Geometry check sheet. Reference: the model listing, model coordinates, mm. Face numbers are marked on the shaded views. A direction names the side the tool comes from. Coordinates: 2 decimals unless noted, no trailing zeros. Order: outer loops, then holes, each group sorted by start corner. A loop starts at its lowest first (then second) coordinate and runs counter-clockwise, first axis right, second up. Notation, with made-up numbers: (17.25, -29.5) - (72.25, -29.5) arc R18 ccw to (72.25, -15.5) - close; hole circle Ø1 at (-39, 16). An arc over 180 degrees is marked (long way). One line per item, written item: value. Start each with the question number.
```python
from build123d import *

# Parameters (mm, degrees)
F0_W     = 84
F0_H     = 68
F1_DEPTH = 50
F4_D     = 20
F5_D     = 20
F5_DEPTH = 50


with BuildPart() as f1:
    # F0 (on Top) → F1 (new body)
    with BuildSketch(Plane.XY):
        Polygon((0, 200), (0, 0), (16, 0), (16, 50), (116, 50), (116, 150), (16, 150), (16, 200), align=None)
        with Locations((58, 100)):
            Rectangle(F0_W, F0_H, mode=Mode.SUBTRACT)
    extrude(amount=F1_DEPTH)

    # F4 (through all)
    with Locations(Plane.YZ.offset(16)):
        with Locations((25, 25), (175, 25)):
            Hole(F4_D / 2)

    # F5
    with Locations(Plane.YZ.offset(116)):
        with Locations((100, 25)):
            Hole(F5_D / 2, depth=F5_DEPTH)


solid = f1.part
```
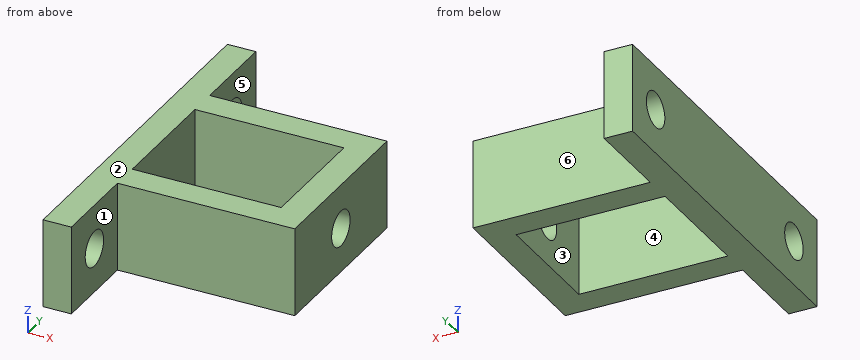
Q1. Cross-section at B-B, the plane x = 91.5. Enter the section's corners in (y, z).
Q2. Material ranges on probe 1 along X at (y, z) = (85, 11); probe 2 along Y at (x, z) = (109.5, 25.5); probe 3 along Z at (x, y) = (107, 100), recorded low to high.
Q3. Cross-section at D-D, the plane y = 100. Enter the section's corners in (x, z).
Q4. Set-up check for the marked faces 1, 2 and 3: record each of +Z, -Z, +X, -X, +Y, -Y from which the full face is reachable in a straight line by a thin tool's end or side.
Q5. Cross-section at A-A, the plane y = 175. Enter the section's corners in (x, z), and give its area (3 significant figures).
Q6. Cross-section at C-C, the plane z = 25. Enter the section's corners in (x, y), and give its area (3 significant figures).
Q7. Gauge pin test, flat ends, axial feed: P1, Ø16, axis at y = 25, z = 25, coming from the +X side; P2, Ø15, axis at y = 15, z = 34.5, coming from the +X side; P3, Ø25, axis at y = 97, z = 17, coming from the -X side; P4, Ø10, axis at x = 39, z = 16, coming from the +Y side. Record the tip position at first contact, or that the pin passes through.
Q8. Release check for a two-part mould opening along Y. For the marked faces 4, 5 and 6 record: released by +Y, released by -Y, zero draft, split by the parting line, or undercut.
Check result:
1. outline: (50, 0) - (66, 0) - (66, 50) - (50, 50) - close; (134, 0) - (150, 0) - (150, 50) - (134, 50) - close
2. probe 1: x = 0 to 16, 100 to 116
2. probe 2: y = 50 to 90.01, 109.99 to 150
2. probe 3: z = 0 to 15, 35 to 50
3. outline: (0, 0) - (16, 0) - (16, 50) - (0, 50) - close; (100, 0) - (116, 0) - (116, 15) - (100, 15) - close; (100, 35) - (116, 35) - (116, 50) - (100, 50) - close
4. face 1: +Z, -Z, +X, -Y
4. face 2: +Z, +X, -X, +Y, -Y
4. face 3: +Z, -Z
5. outline: (0, 0) - (16, 0) - (16, 15) - (0, 15) - close; (0, 35) - (16, 35) - (16, 50) - (0, 50) - close
5. area: 480 mm2
6. outline: (0, 0) - (16, 0) - (16, 15) - (0, 15) - close; (0, 35) - (16, 35) - (16, 50) - (116, 50) - (116, 90) - (100, 90) - (100, 66) - (16, 66) - (16, 134) - (100, 134) - (100, 110) - (116, 110) - (116, 150) - (16, 150) - (16, 165) - (0, 165) - close; (0, 185) - (16, 185) - (16, 200) - (0, 200) - close
6. area: 6,530 mm2
7. P1: passes through
7. P2: stops at x = 16
7. P3: stops at x = 0
7. P4: stops at y = 150
8. face 4: undercut
8. face 5: zero draft
8. face 6: released by +Y
